Could you check a few things on this model? Use its own coordinates, in mm. A direction names the side the tool comes from. Coordinates: 2 decimals unless noted, no trailing zeros. Loops run counter-clockwise (first coordinate to the right, second up) from the corner with the lowest first, then second, coordinate; pieces in that order, holes last. Notation, with made-up numbers: (28, 44.5) -> (37, 44.5) arc R29 ccw to (37, 66.5) -> close; hole circle Ø7 at (-34.75, 71). An arc over 180 degrees is marked (long way). One line per question, with ' | ' between items.
```python
from build123d import *

# Parameters (mm, degrees)
F1_DEPTH  = 3
F3_W      = 3
F3_H      = 177.7333333333
F3_H_2    = 157.7333333333
F3_H_3    = 127.0666666667
F3_H_4    = 96.4
F3_H_5    = 65.7333333333
F4_DEPTH  = 1800
F7_DEPTH  = 3
F10_DEPTH = 3
F11_W     = 2100
F11_H     = 1800
F12_DEPTH = 2
F14_DEPTH = 3


with BuildPart() as f1:
    # F0 (on Front) → F1 (new body)
    with BuildSketch(Plane.XZ):
        Polygon((-1050, -314.938241453), (0, -314.938241453), (1050, -314.938241453), (1050, -254.938241453), (958, -242.6715747864), (955, -242.2715747864), (808, -222.6715747864), (805, -222.2715747864), (578, -192.0049081197), (575, -191.6049081197), (348, -161.338241453), (345, -160.938241453), (118, -130.6715747864), (115, -130.2715747864), (0, -114.938241453), (-115, -130.2715747864), (-118, -130.6715747864), (-345, -160.938241453), (-348, -161.338241453), (-575, -191.6049081197), (-578, -192.0049081197), (-805, -222.2715747864), (-808, -222.6715747864), (-955, -242.2715747864), (-958, -242.6715747864), (-1050, -254.938241453), align=None)
        Polygon((-958, -64.938241453), (-958, -242.6715747864), (-955, -242.2715747864), (-955, -64.938241453), align=None)
        Polygon((955, -242.2715747864), (958, -242.6715747864), (958, -64.938241453), (955, -64.938241453), align=None)
        Polygon((-808, -64.938241453), (-808, -222.6715747864), (-805, -222.2715747864), (-805, -64.938241453), align=None)
        Polygon((805, -222.2715747864), (808, -222.6715747864), (808, -64.938241453), (805, -64.938241453), align=None)
        Polygon((-578, -64.938241453), (-578, -192.0049081197), (-575, -191.6049081197), (-575, -64.938241453), align=None)
        Polygon((575, -191.6049081197), (578, -192.0049081197), (578, -64.938241453), (575, -64.938241453), align=None)
        Polygon((-348, -64.938241453), (-348, -161.338241453), (-345, -160.938241453), (-345, -64.938241453), align=None)
        Polygon((345, -160.938241453), (348, -161.338241453), (348, -64.938241453), (345, -64.938241453), align=None)
        Polygon((-118, -64.938241453), (-118, -130.6715747864), (-115, -130.2715747864), (-115, -64.938241453), align=None)
        Polygon((115, -130.2715747864), (118, -130.6715747864), (118, -64.938241453), (115, -64.938241453), align=None)
    extrude(amount=F1_DEPTH)

    # F3 (on offset) → F4 (join)
    with BuildSketch(Plane.XZ.offset(603)):
        with Locations((-956.5, -153.8049081197)):
            Rectangle(F3_W, F3_H)
        with Locations((-806.5, -143.8049081197)):
            Rectangle(F3_W, F3_H_2)
        with Locations((-576.5, -128.4715747864)):
            Rectangle(F3_W, F3_H_3)
        with Locations((-346.5, -113.138241453)):
            Rectangle(F3_W, F3_H_4)
        with Locations((-116.5, -97.8049081197)):
            Rectangle(F3_W, F3_H_5)
        with Locations((346.5, -113.138241453)):
            Rectangle(F3_W, F3_H_4)
        with Locations((576.5, -128.4715747864)):
            Rectangle(F3_W, F3_H_3)
        with Locations((806.5, -143.8049081197)):
            Rectangle(F3_W, F3_H_2)
        with Locations((116.5, -97.8049081197)):
            Rectangle(F3_W, F3_H_5)
        with Locations((956.5, -153.8049081197)):
            Rectangle(F3_W, F3_H)
    extrude(amount=-F4_DEPTH)

    # F6 (on offset) → F7 (join)
    with BuildSketch(Plane.XZ.offset(-597)):
        Polygon((1050, -254.938241453), (0, -116.9179081917), (-1050, -254.938241453), (-1050, -314.938241453), (0, -314.938241453), (1050, -314.938241453), align=None)
    extrude(amount=F7_DEPTH)

    # F9 (on offset) → F10 (join)
    with BuildSketch(Plane.XZ.offset(-1197)):
        Polygon((1050, -254.938241453), (0, -114.938241453), (-1050, -254.938241453), (-1050, -314.938241453), (0, -314.938241453), (1050, -314.938241453), align=None)
    extrude(amount=F10_DEPTH)

    # F11 (on face) → F12 (join)
    with BuildSketch(Plane.XY.offset(-64.938241453)):
        with Locations((0, 297)):
            Rectangle(F11_W, F11_H)
    extrude(amount=F12_DEPTH)

    # F13 (on offset) → F14 (join)
    with BuildSketch(Plane.XZ.offset(603)):
        Polygon((1050, -254.938241453), (0, -114.938241453), (-1050, -254.938241453), (-1050, -314.938241453), (0, -314.938241453), (1050, -314.938241453), align=None)
    extrude(amount=F14_DEPTH)


solid = f1.part
```
Q1. Please list where these lines run through material, in increasing order: L1, parallel to Y at x = 626.5, z = -296; L2, parallel to X at y = 948.5, z = -191; L3, parallel to Z at x = 557, y = 334.5. Write a range as [from, to].
Values follow:
L1: y = [-606, -603], [-3, 0], [594, 597], [1194, 1197] | L2: x = [-958, -955], [-808, -805], [-578, -575], [575, 578], [805, 808], [955, 958] | L3: z = [-64.94, -62.94]
Q2. For faces 4 (the face through (-15, 310, -62.938)), 5 (the face through (-15, -3, -236)), which set-ups out of +Z, -Z, +X, -X, +Y, -Y let a thin tool reach every point of the face, with its end or its side?
Values follow:
face 4: +Z, +X, -X, +Y, -Y | face 5: -Z
Q3. Imagine slicing it at A-A on z = -285. Write out the boundary of the cut face in (x, y).
Values follow:
outline: (-1050, -606) -> (1050, -606) -> (1050, -603) -> (-1050, -603) -> close; (-1050, -3) -> (1050, -3) -> (1050, 0) -> (-1050, 0) -> close; (-1050, 594) -> (1050, 594) -> (1050, 597) -> (-1050, 597) -> close; (-1050, 1194) -> (1050, 1194) -> (1050, 1197) -> (-1050, 1197) -> close
Q4. We'd pull the mould along Y, two halves only. Please class faces 1 (the face through (-15, -606, -236)), 2 (the face through (-15, 594, -237)), 3 (the face through (808, 284, -145)): released by +Y, released by -Y, zero draft, split by the parting line, or undercut.
Values follow:
face 1: released by -Y | face 2: undercut | face 3: zero draft
Q5. For pin 1 (12 mm diameter, centred on x = 784.5, y = -411, fed in from -Z); pin 2 (0.9 mm diameter, centred on x = 576.5, y = 301, fed in from -Z); pin 3 (1.5 mm diameter, centred on x = -806, y = 771, fed in from -Z), each with a flat end and sliding along its axis, tell me the tip position at first contact or that it passes through.
Values follow:
pin 1: stops at z = -64.94 | pin 2: stops at z = -192 | pin 3: stops at z = -222.67
Q6. Imagine slicing it at B-B on x = -268. Write out the boundary of the cut face in (y, z), plus the area to 3 significant figures.
Values follow:
outline: (-606, -314.94) -> (-603, -314.94) -> (-603, -150.67) -> (-606, -150.67) -> close; (-603, -64.94) -> (1197, -64.94) -> (1197, -62.94) -> (-603, -62.94) -> close; (-3, -314.94) -> (0, -314.94) -> (0, -150.67) -> (-3, -150.67) -> close; (594, -314.94) -> (597, -314.94) -> (597, -152.15) -> (594, -152.15) -> close; (1194, -314.94) -> (1197, -314.94) -> (1197, -150.67) -> (1194, -150.67) -> close | area: 5,570 mm2
